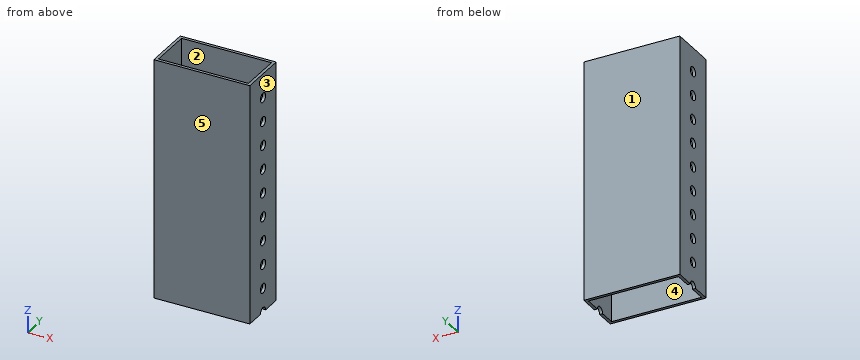
from build123d import *

# Parameters (mm, degrees)
SKETCH1_W           = 50.8
SKETCH1_H           = 25.4
SKETCH1_W_2         = 47.625
SKETCH1_H_2         = 22.225
BOSS_EXTRUDE1_DEPTH = 127
SKETCH2_R           = 2.4892
CUT_EXTRUDE1_DEPTH  = 51.8


with BuildPart() as part:
    # Sketch1 → Boss-Extrude1 (new body)
    with BuildSketch(Plane.XY):
        with Locations((25.4, 12.7)):
            Rectangle(SKETCH1_W, SKETCH1_H)
        with Locations((25.4, 12.7)):
            Rectangle(SKETCH1_W_2, SKETCH1_H_2, mode=Mode.SUBTRACT)
    extrude(amount=BOSS_EXTRUDE1_DEPTH)

    # Sketch2 → Cut-Extrude1 (cut, through all)
    with BuildSketch(Plane(origin=(50.8, 0, 0), x_dir=(0, 0, -1), z_dir=(1, 0, 0))):
        with Locations((-114.3, 12.7)):
            Circle(SKETCH2_R)
        with Locations((-101.6, 12.7)):
            Circle(SKETCH2_R)
        with Locations((-88.9, 12.7)):
            Circle(SKETCH2_R)
        with Locations((-76.2, 12.7)):
            Circle(SKETCH2_R)
        with Locations((-63.5, 12.7)):
            Circle(SKETCH2_R)
        with Locations((-50.8, 12.7)):
            Circle(SKETCH2_R)
        with Locations((-38.1, 12.7)):
            Circle(SKETCH2_R)
        with Locations((-25.4, 12.7)):
            Circle(SKETCH2_R)
        with Locations((-12.7, 12.7)):
            Circle(SKETCH2_R)
        with Locations((0, 12.7)):
            Circle(SKETCH2_R)
        with Locations((12.7, 12.7)):
            Circle(SKETCH2_R)
    extrude(amount=-CUT_EXTRUDE1_DEPTH, mode=Mode.SUBTRACT)


solid = part.part
Source: CAD feature listing. Evaluate the final solid. Frame: model axes, mm. Face numbers are marked on the shaded views. A direction names the side the tool comes from. Round coordinates to 2 decimals unless told otherwise and drop trailing zeros. Order: outer loops, then holes, each group sorted by start corner. A loop starts at its lowest first (then second) coordinate and runs counter-clockwise, first axis right, second up. Notation, with made-up numbers: (70, 40) - (99, 40) arc R25 ccw to (99, 56) - close; hole circle Ø1 at (22.25, -32.75). An arc over 180 degrees is marked (long way). Use a Markdown table: item, result. Add a question column.
1. Line query: probe 1 along X at (y, z) = (9.5, 120.5); probe 2 along Y at (x, z) = (42.5, 100); probe 3 along Y at (x, z) = (0.8, 114.3). Output: solid intervals per line, ascending.
2. Set-up query: the marked faces 1 and 2. Return all of +Z, -Z, +X, -X, +Y, -Y with unobstructed straight access to the full face (end or side cutting, diameter ignored); none if empty.
3. Mould query, pull axis Y, two halves, no side actions, for the marked faces 3, 4 and 5. Classes: +Y half, -Y half, draft (parallel to the pull), parting line (faces both ways), or undercut.
4. Section query B-B (z = 8). Return the cut outline in (x, y).
5. Section query C-C (y = 20). Return the cut outline in (x, z), then the cut area to 3 significant figures.
6. Section query A-A (x = 43). Return the cut outline in (y, z).
7. Section query D-D (z = 88.9). Return the cut outline in (x, y), then the cut area to 3 significant figures.
Derived:
| question | item | result |
|---|---|---|
| 1 | probe 1 | 0 to 1.59, 49.21 to 50.8 |
| 1 | probe 2 | 0 to 1.59, 23.81 to 25.4 |
| 1 | probe 3 | 0 to 10.21, 15.19 to 25.4 |
| 2 | face 1 | +Z, -Z, +X, -X, +Y |
| 2 | face 2 | +Z, -Z |
| 3 | face 3 | draft |
| 3 | face 4 | undercut |
| 3 | face 5 | -Y half |
| 4 | outline | (0, 0) - (50.8, 0) - (50.8, 25.4) - (0, 25.4) - close; hole (1.59, 1.59) - (49.21, 1.59) - (49.21, 23.81) - (1.59, 23.81) - close |
| 5 | outline | (0, 0) - (1.59, 0) - (1.59, 127) - (0, 127) - close; (49.21, 0) - (50.8, 0) - (50.8, 127) - (49.21, 127) - close |
| 5 | area | 403 mm2 |
| 6 | outline | (0, 0) - (1.59, 0) - (1.59, 127) - (0, 127) - close; (23.81, 0) - (25.4, 0) - (25.4, 127) - (23.81, 127) - close |
| 7 | outline | (0, 0) - (50.8, 0) - (50.8, 10.21) - (49.21, 10.21) - (49.21, 1.59) - (1.59, 1.59) - (1.59, 10.21) - (0, 10.21) - close; (0, 15.19) - (1.59, 15.19) - (1.59, 23.81) - (49.21, 23.81) - (49.21, 15.19) - (50.8, 15.19) - (50.8, 25.4) - (0, 25.4) - close |
| 7 | area | 216 mm2 |
